from build123d import *

# Parameters (mm, degrees)
SKETCH1_W                                     = 330.2
SKETCH1_H                                     = 127
MAIN_PLATE_SIZE_DEPTH                         = 6.35
SKETCH2_R                                     = 9.525
SKETCH2_R_2                                   = 1.778
BOTTOM_SHAFT_MOUNTING_HOLES_DEPTH             = 354.83804558
SKETCH3_R                                     = 6.35
SKETCH3_R_2                                   = 1.778
TOP_BATTERY_BOX_MOUNTING_HOLES_DEPTH          = 354.83804558
THIS_IS_TO_MATCH_THE_IDIOTIC_DESIGN_OF_B_SIZE = 6.35
THIS_IS_TO_MATCH_THE_IDIOTIC_DESIGN_2_R       = 10
SKETCH4_R                                     = 2.5
F_20MM_EXTRUSION_MOUNT_DEPTH                  = 354.83804558


with BuildPart() as part:
    # Sketch1 → Main Plate Size (new body)
    with BuildSketch(Plane(origin=(0, 0, 0), x_dir=(0, 0, -1), z_dir=(1, 0, 0))):
        with Locations((165.1, 63.5)):
            Rectangle(SKETCH1_W, SKETCH1_H)
    extrude(amount=MAIN_PLATE_SIZE_DEPTH)

    # Sketch2 → Bottom Shaft Mounting Holes (cut, through all)
    with BuildSketch(Plane(origin=(6.35, 0, 0), x_dir=(0, 0, -1), z_dir=(1, 0, 0))):
        with BuildLine():
            Line((134.1120127, 20.8026), (0, 20.8026))
            Line((0, 20.8026), (0, 0))
            Line((0, 0), (159.512000023, 0))
            ThreePointArc((159.512000023, 0), (143.096249024, 5.864358018), (134.1120127, 20.8026))
        make_face()
        with BuildLine():
            ThreePointArc((184.9119873, 20.8026), (175.927750994, 5.864358033), (159.512000023, 0))
            Line((159.512000023, 0), (177.8, 0))
            Line((177.8, 0), (330.2, 0))
            Line((330.2, 0), (330.2, 20.8026))
            Line((330.2, 20.8026), (184.9119873, 20.8026))
        make_face()
        with Locations((159.512, 23.8252)):
            Circle(SKETCH2_R)
        with Locations((159.512, 4.7752)):
            Circle(SKETCH2_R_2)
        with Locations((178.562, 23.8252)):
            Circle(SKETCH2_R_2)
        with Locations((159.512, 42.8752)):
            Circle(SKETCH2_R_2)
        with Locations((140.462, 23.8252)):
            Circle(SKETCH2_R_2)
    extrude(amount=-BOTTOM_SHAFT_MOUNTING_HOLES_DEPTH, mode=Mode.SUBTRACT)

    # Sketch3 → Top Battery Box Mounting Holes (cut, through all)
    with BuildSketch(Plane(origin=(6.35, 0, 0), x_dir=(0, 0, -1), z_dir=(1, 0, 0))):
        with Locations((159.512, 106.5022)):
            Circle(SKETCH3_R)
        with Locations((149.733, 106.5022)):
            Circle(SKETCH3_R_2)
        with Locations((159.512, 116.2812)):
            Circle(SKETCH3_R_2)
        with Locations((169.291, 106.5022)):
            Circle(SKETCH3_R_2)
        with Locations((159.512, 96.7232)):
            Circle(SKETCH3_R_2)
    extrude(amount=-TOP_BATTERY_BOX_MOUNTING_HOLES_DEPTH, mode=Mode.SUBTRACT)

    # This is to match the idiotic Design of B
    # the kernel refuses this chamfer: 6.35 mm, written as the material it adds along each edge
    with BuildSketch(Plane(origin=(6.35, 20.8026, -134.1120127), x_dir=(0, -0.9387383646661532, -0.34463064678568023), z_dir=(-1, 0, 0))) as this_is_to_match_the_idiotic_design_of_b_piece_1:
        with BuildLine():
            Line((7.921958409, 0), (-THIS_IS_TO_MATCH_THE_IDIOTIC_DESIGN_OF_B_SIZE * 0.344630646786, THIS_IS_TO_MATCH_THE_IDIOTIC_DESIGN_OF_B_SIZE * 0.938738364666))
            Line((-THIS_IS_TO_MATCH_THE_IDIOTIC_DESIGN_OF_B_SIZE * 0.344630646786, THIS_IS_TO_MATCH_THE_IDIOTIC_DESIGN_OF_B_SIZE * 0.938738364666), (0, 0))
            ThreePointArc((0, 0), (4.071959946, 0.304342453), (7.921958409, 0))
        make_face()
    extrude(amount=6.35)
    with BuildSketch(Plane(origin=(6.35, 20.8026, -184.9119873), x_dir=(0, -0.9387383646661542, 0.34463064678567756), z_dir=(-1, 0, 0))) as this_is_to_match_the_idiotic_design_of_b_piece_2:
        with BuildLine():
            Line((7.921958409, 0), (-THIS_IS_TO_MATCH_THE_IDIOTIC_DESIGN_OF_B_SIZE * 0.344630646786, -THIS_IS_TO_MATCH_THE_IDIOTIC_DESIGN_OF_B_SIZE * 0.938738364666))
            Line((-THIS_IS_TO_MATCH_THE_IDIOTIC_DESIGN_OF_B_SIZE * 0.344630646786, -THIS_IS_TO_MATCH_THE_IDIOTIC_DESIGN_OF_B_SIZE * 0.938738364666), (0, 0))
            ThreePointArc((0, 0), (4.071959946, -0.304342453), (7.921958409, 0))
        make_face()
    extrude(amount=6.35)

    # This is to match the idiotic Design  2
    this_is_to_match_the_idiotic_design_2_edges = [part.edges().sort_by_distance(p)[0] for p in [
        (3.175, 13.365953718, -136.84216235),
        (3.175, 13.365953718, -182.18183765),
        (3.175, 20.8026, -191.2619873),
        (3.175, 20.8026, -127.7620127),
    ]]
    fillet(this_is_to_match_the_idiotic_design_2_edges, radius=THIS_IS_TO_MATCH_THE_IDIOTIC_DESIGN_2_R)

    # Sketch4 → 20mm Extrusion Mount (cut, through all)
    with BuildSketch(Plane(origin=(6.35, 0, 0), x_dir=(0, 0, -1), z_dir=(1, 0, 0))):
        with Locations((10, 97.0026)):
            Circle(SKETCH4_R)
    extrude(amount=-F_20MM_EXTRUSION_MOUNT_DEPTH, mode=Mode.SUBTRACT)


solid = part.part
Input: part model. Units: mm. Frame: model coordinates. A direction names the side the tool comes from. Coordinates: 2 decimals unless noted, no trailing zeros. Order: outer loops, then holes, each group sorted by start corner. A loop starts at its lowest first (then second) coordinate and runs counter-clockwise, first axis right, second up. Notation, with made-up numbers: M 75.5,-4 L 117.5,-4 A21 ccw 117.5,32 Z; hole C 45,-40 d2. An arc over 180 degrees is marked long. Write item = value, one per line. Start each with the question number.
(1) First-contact query: P1, Ø3, axis at y = 42.88, z = -159.51, coming from the -X side; P2, Ø3, axis at x = 2.5, z = -278, coming from the -Y side. Flat tips, straight axial feed; report the tip coordinate or a pass-through.
(2) Section B-B on z = -74. Output: boundary loops of the cut face in (x, y).
(3) Pull-direction query (Y, two-part tool) for faces 4 (the flat face through (3, 127, -163)), 5 (the cylindrical face through (3.2, 102.6, -154.5)), 6 (the flat face through (3, 73, 0)); classes: released by +Y, released by -Y, zero draft, split by the parting line, or undercut.
(4) Reachability of faces 1 (the flat face through (3, 20.803, -63)), 2 (the flat face through (3, 73, -330.2)), 3 (the flat face through (3, 20.803, -263)) from +Z, -Z, +X, -X, +Y, -Y: full face, straight path, thin tool, end or side. Return the list, or none.
(5) Section A-A on x = 1.25. Give the number of separate pieces and of enclosed holes in the cut face, and give its area (3 significant figures).
(6) Line query: line 1 along Y through (x, z) = (1.25, -168); line 2 along Z through (x, y) = (4.75, 106); line 3 along Y through (x, z) = (0.75, -211). Output: solid intervals per line, ascending. Write a range as [from, to].
Result set:
q1.P1 = through
q1.P2 = 20.8
q2.outline = M 0,20.8 L 6.35,20.8 L 6.35,127 L 0,127 Z
q3.face_4 = released by +Y
q3.face_5 = undercut
q3.face_6 = zero draft
q4.face_1 = +Z, +X, -X, -Y
q4.face_2 = -Z, +X, -X, +Y, -Y
q4.face_3 = -Z, +X, -X, -Y
q5.separate_pieces = 1
q5.enclosed_holes = 11
q5.area = 35,400 mm²
q6.line_1 = [1.43, 19.5], [28.15, 105.28], [107.72, 127]
q6.line_2 = [-330.2, -171], [-167.59, -165.84], [-153.18, -151.44], [-148.03, 0]
q6.line_3 = [20.8, 127]
